The listing builds one solid part. Answer for the finished solid, in the listing's coordinates (mm). A direction names the side the tool comes from. Coordinates: 2 decimals unless noted, no trailing zeros. Write each loop counter-clockwise with the first axis right and the second up, starting at its lowest first coordinate (ties: lowest second). Pieces come first, ordered by that corner, then holes.
(1) The part is cut by section C-C on y = -11.5. Determine the outline of the cut face in (x, z), plus the area to 3 significant figures.
(2) For a pull along Z with two mould halves and no side action, classify faces 6 (the flat face through (-4, -10, 10)), 7 (the flat face through (-4, -10, 0)), 8 (the flat face through (7.071, 10, 5)), 9 (the flat face through (0.9, -12, 6.4)) as +Z half, -Z half, draft (parallel to the pull), parting line (faces both ways), or undercut.
(3) Given P1, Ø4.5, axis at y = 11.5, z = 4.5, coming from the -X side; P2, Ø3, axis at x = 6.5, z = 3, coming from the +Y side; P3, Ø1.5, axis at x = 5.5, z = 3, coming from the +Y side, each flat-ended and moving along its own axis, determine where each tip first touches the part or whether it passes through.
(4) Straight lines are drawn through the part: line 1 (X direction, y = 9, z = 7.5); line 2 (Z direction, x = 0, y = -15.1); line 3 (Y direction, x = -8.95, z = 5). For each, find the intervals that lie inside material, in ascending order.
(5) Which of the six approach directions +Z, -Z, +X, -X, +Y, -Y give full straight-line access (tool end or side, diameter ignored) to faces 1 (the cylindrical face through (-2.08, -10.91, 5.09)), 2 (the cylindrical face through (7.641, 17.177, 4.93)), 3 (the flat face through (12.778, 15, 5)), 4 (the flat face through (15, -13, 5)), 5 (the flat face through (-12.778, 15, 5))?
(6) The part is cut by section B-B on y = 10. Determine the outline of the cut face in (x, z), plus the area to 3 significant figures.
(7) The part is cut by section A-A on x = 0. Determine the outline of the cut face in (y, z).
Autodesk Inventor part; units mm, degrees
ref_plane "YZ Plane" through (0, 0, 0) normal (1, 0, 0) x (0, 1, 0)
ref_plane "XZ Plane" through (0, 0, 0) normal (0, 1, 0) x (-1, 0, 0)
ref_plane "XY Plane" through (0, 0, 0) normal (0, 0, 1) x (1, 0, 0)
sketch "Sketch1" plane through (0, 0, 0) normal (0, 0, 1) x (1, 0, 0)
  line L0 (0, 0) -> (15.5887, 0) construction
  line L1 (0, 0) -> (20, 0) construction
  line L2 (15, -11) -> (15, -16)
  line L3 (15, -16) -> (-15, -16)
  line L4 (-15, -16) -> (-15, -11)
  line L5 (-15, -11) -> (-10.198, -11)
  arc A0 (-10.6066, 10.6066) -> (-10.198, -11) centre (0, 0) ccw
  arc A1 (10.198, -11) -> (10.6066, 10.6066) centre (0, 0) ccw
  line L6 (15, -11) -> (10.198, -11)
  arc A2 (-7.0711, 7.0711) -> (7.0711, 7.0711) centre (0, 0) ccw
  line L7 (10.6066, 10.6066) -> (7.0711, 7.0711)
  line L8 (-7.0711, 7.0711) -> (-10.6066, 10.6066)
  dimension "d6" = 5
  dimension "d7" = 30
  dimension "d35" = 20
extrude "Extrusion1" add sketch "Sketch1" along normal blind 10
sketch "Sketch2" plane through (-15, -16, 0) normal (0, -1, 0) x (1, 0, 0)
  line L0 (0, 10) -> (30, 10)
  line L1 (30, 10) -> (25.198, 10)
  line L2 (0, 0) -> (30, 0)
  circle A0 centre (15, 5) radius 1.5
  point P0 (15, 0)
  dimension "d10" = 3
extrude "Extrusion2" cut sketch "Sketch2" against normal blind 24.75
sketch "Sketch3" plane through (10.198, -11, 0) normal (0, 1, 0) x (1, 0, 0)
  line L0 (4.802, 0) -> (0, 0)
  line L1 (-20.3961, -10) -> (-25.198, -10)
  line L2 (-20.3961, 0) -> (-25.198, 0)
  line L3 (4.802, -10) -> (0, -10)
  circle A0 centre (-10.198, -5) radius 2.0833
  point P0 (-10.198, 0)
sketch "Sketch4" plane through (0, 0, 0) normal (0, 0, -1) x (-1, 0, 0)
  point P0 (0, 0)
extrude "Extrusion3" cut sketch "Sketch3" against normal blind 1
sketch "Sketch5" plane through (10.198, -11, 0) normal (0, -1, 0) x (1, 0, 0)
  circle A0 centre (-10.198, 5) radius 1.5
  circle A1 centre (-10.198, 5) radius 2.0833
  circle A2 centre (-10.198, 5) radius 2.0833
  point P0 (-10.198, 0)
  point P1 (-10.198, 6.5)
  point P2 (-10.198, 3.5)
  point P3 (-10.198, 2.9167)
  point P4 (-10.198, 7.0833)
  point P5 (-10.198, 2.9167)
extrude "Extrusion4" cut sketch "Sketch5" against normal blind 1.5 contours A0 | A1
fillet "Fillet1" radius 2 1 edges at (-10.198, -11, 5)
fillet "Fillet2" radius 2 1 edges at (10.198, -11, 5)
sketch "Sketch6" plane through (0, 0, 10) normal (0, 0, 1) x (1, 0, 0)
  line L0 (-7.7782, 7.7782) -> (-10.6066, 10.6066)
  line L1 (-12.7782, 17.7782) -> (-12.7782, 7.8561)
  arc A0 (-10.6066, 10.6066) -> (-12.7255, -7.9412) centre (0, 0) ccw
  arc A1 (-7.0711, 7.0711) -> (7.0711, 7.0711) centre (0, 0) ccw construction
  line L2 (-7.0711, 7.0711) -> (-10.6066, 10.6066)
  line L3 (-7.0711, 7.0711) -> (-7.0711, 17.7782)
  line L4 (-12.7782, 17.7782) -> (-7.0711, 17.7782)
extrude "Extrusion5" add sketch "Sketch6" against normal blind 10
sketch "Sketch7" plane through (0, 0, 10) normal (0, 0, 1) x (1, 0, 0)
  line L0 (12.7782, 17.7782) -> (12.7782, 7.8561)
  arc A0 (12.7255, -7.9412) -> (10.6066, 10.6066) centre (0, 0) ccw
  arc A1 (-7.7782, 7.7782) -> (7.7782, 7.7782) centre (0, 0) ccw
  arc A2 (-7.0711, 7.0711) -> (7.0711, 7.0711) centre (0, 0) ccw
  line L1 (7.0711, 7.0711) -> (7.0711, 17.7782)
  line L2 (12.7782, 17.7782) -> (7.0711, 17.7782)
  line L3 (7.0711, 7.0711) -> (12.7782, 7.8561)
extrude "Extrusion6" add sketch "Sketch7" against normal blind 10
sketch "Sketch8" plane through (12.7782, 7.8561, 10) normal (1, 0, 0) x (0, 0, -1)
  line L0 (0, 9.9221) -> (0, 0) construction
  line L1 (10, -0.0779) -> (0, -0.0779) construction
  line L2 (0, 9.9221) -> (10, -0.0779) construction
  line L3 (0, 9.9221) -> (10, 9.9221) construction
  line L4 (10, 9.9221) -> (0, -0.0779) construction
  circle A0 centre (5, 4.9221) radius 2
  point P0 (10, -7.8561)
  dimension "d28" = 4
extrude "Extrusion7" cut sketch "Sketch8" against normal blind 36
fillet "Fillet9" radius 2 1 edges at (-7.0711, 17.7782, 5)
fillet "Fillet10" radius 2 1 edges at (7.0711, 17.7782, 5)
properties part number "buisClip"
Model answer:
1. outline: (-15, 0) - (15, 0) - (15, 10) - (-15, 10) - close; hole circle Ø4.17 at (0, 5)
1. area: 286 mm2
2. face 6: +Z half
2. face 7: -Z half
2. face 8: draft
2. face 9: undercut
3. P1: stops at x = -12.78
3. P2: stops at y = 17.47
3. P3: stops at y = -7.81
4. line 1: x = -12.78 to -7.07, 7.07 to 12.78
4. line 2: z = 0 to 3.5, 6.5 to 10
4. line 3: y = -16 to -4.46, 4.46 to 10.78, 14.78 to 17.77
5. face 1: +Y
5. face 2: +Z, -Z, +Y
5. face 3: +Z, -Z, +X, +Y
5. face 4: +Z, -Z, +X, +Y, -Y
5. face 5: +Z, -Z, -X, +Y
6. outline: (-12.78, 0) - (-7.07, 0) - (-7.07, 10) - (-12.78, 10) - close; (7.07, 0) - (12.78, 0) - (12.78, 10) - (7.07, 10) - close
6. area: 114 mm2
7. outline: (-16, 0) - (-10, 0) - (-10, 2.92) - (-12, 2.92) - (-12, 3.5) - (-16, 3.5) - close; (-16, 6.5) - (-12, 6.5) - (-12, 7.08) - (-10, 7.08) - (-10, 10) - (-16, 10) - close
